Model file for the job. Use its own axes, mm. A direction names the side the tool comes from. Give positions to 0.01 mm unless a question says otherwise; leave off trailing zeros. Write each loop counter-clockwise with the first axis right and the second up, starting at its lowest first coordinate (ties: lowest second). Pieces come first, ordered by that corner, then holes. Notation, with made-up numbers: (73, 44) - (95, 44) arc R19 ccw to (95, 70) - close; hole circle Ø7 at (5, 52.5). An arc over 180 degrees is marked (long way). Use a Markdown table: item, result. Add a question column.
```python
from build123d import *

# Parameters (mm, degrees)
F1_DEPTH = 9
F2_R     = 5.5
F3_DEPTH = 51
F4_R     = 2.1
F5_DEPTH = 25
F6_R     = 5
F7_DEPTH = 25
F8_W     = 95
F8_H     = 11
F9_DEPTH = 25
F10_SIZE = 5
F11_SIZE = 2.1
F12_SIZE = 0.5


with BuildPart() as f1:
    # F0 (on Front) → F1 (new body, symmetric)
    with BuildSketch(Plane.XZ):
        Polygon((-245, 13.5), (-245, -37.5), (245, -37.5), (245, 13.5), (150, 13.5), (150, 37.5), (-150, 37.5), (-150, 13.5), align=None)
    extrude(amount=F1_DEPTH, both=True)

    # F2 (on face) → F3 (cut, through all)
    with BuildSketch(Plane(origin=(0, 0, -37.5), x_dir=(1, 0, 0), z_dir=(0, 0, -1))):
        with Locations((235, 0)):
            Circle(F2_R)
        with Locations((165, 0)):
            Circle(F2_R)
        with Locations((-165, 0)):
            Circle(F2_R)
        with Locations((-235, 0)):
            Circle(F2_R)
    extrude(amount=-F3_DEPTH, mode=Mode.SUBTRACT)

    # F4 (on face) → F5 (cut)
    with BuildSketch(Plane.XY.offset(37.5)):
        with Locations((-115, 0)):
            Circle(F4_R)
        with Locations((-55, 0)):
            Circle(F4_R)
        with Locations((5, 0)):
            Circle(F4_R)
        with Locations((65, 0)):
            Circle(F4_R)
        with Locations((125, 0)):
            Circle(F4_R)
    extrude(amount=-F5_DEPTH, mode=Mode.SUBTRACT)

    # F6 (on face) → F7 (cut)
    with BuildSketch(Plane.XY.offset(13.5)):
        with Locations((-200, 0)):
            Circle(F6_R)
        with Locations((200, 0)):
            Circle(F6_R)
    extrude(amount=-F7_DEPTH, mode=Mode.SUBTRACT)

    # F8 (on face) → F9 (cut)
    with BuildSketch(Plane.XZ.offset(9)):
        with Locations((-197.5, -32)):
            Rectangle(F8_W, F8_H)
        with Locations((197.5, -32)):
            Rectangle(F8_W, F8_H)
    extrude(amount=-F9_DEPTH, mode=Mode.SUBTRACT)

    # F10
    f10_edges = [f1.edges().sort_by_distance(p)[0] for p in [
        (-205, 0, -11.5),
        (195, 0, -11.5),
    ]]
    chamfer(f10_edges, length=F10_SIZE)

    # F11
    f11_edges = [f1.edges().sort_by_distance(p)[0] for p in [
        (122.9, 0, 12.5),
        (62.9, 0, 12.5),
        (2.9, 0, 12.5),
        (-57.1, 0, 12.5),
        (-117.1, 0, 12.5),
    ]]
    chamfer(f11_edges, length=F11_SIZE)

    # F12
    f12_edges = [f1.edges().sort_by_distance(p)[0] for p in [
        (-170.5, 0, -26.5),
        (-159.5, 0, -6.5),
        (-170.5, 0, 13.5),
        (-240.5, 0, -26.5),
        (-229.5, 0, -6.5),
        (-240.5, 0, 13.5),
        (-205, 0, 13.5),
        (-117.1, 0, 37.5),
        (-57.1, 0, 37.5),
        (2.9, 0, 37.5),
        (62.9, 0, 37.5),
        (122.9, 0, 37.5),
        (159.5, 0, -26.5),
        (170.5, 0, -6.5),
        (159.5, 0, 13.5),
        (229.5, 0, -26.5),
        (240.5, 0, -6.5),
        (229.5, 0, 13.5),
        (195, 0, 13.5),
    ]]
    chamfer(f12_edges, length=F12_SIZE)


solid = f1.part
```
(1) Band-saw the part on A-A (x = -165). Write the cut outline in (y, z), then the cut area to 4 significant figures.
(2) Which spindle directions (+Z, -Z, +X, -X, +Y, -Y) get a long thin tool onto all of the face, cutting with end or side? Do faces 1 (the cylindrical face through (204.77, 1.5, 3.39)), 2 (the flat face through (198, 6, 13.5)), 3 (the flat face through (-150, 0, -32)). Say none if no direction does.
(3) Flat gauge pins, fed straight in: pin 1 (9 mm diameter, centred on y = 4, z = 27.5, fed in from +X); pin 2 (6 mm diameter, centred on x = -164, y = 3.5, fed in from +Z); pin 3 (9 mm diameter, centred on y = -4.5, z = 26.5, fed in from -X). Where does each tip first touch, or does it go through?
(4) Probe probe 1 along X at (y, z) = (0, -18); probe 2 along Y at (x, z) = (-235, 2); probe 3 along Y at (x, z) = (65, 31.75). List the from-to ranges inside material, lowest first. Write a range as [from, to].
(5) Band-saw the part on B-B (z = 28.5). Write the cut outline in (x, y).
(6) Band-saw the part on C-C (z = -31.5). Write the cut outline in (x, y), then the cut area to 3 significant figures.
(7) Two-plate mould, pull along X, no slides. Class faces 4 (the cylindrical face through (159.505, -0.242, -6.773)), 5 (the flat face through (-3, -9, 1)), 6 (the flat face through (-150, 0, 26)): +X half, -X half, draft (parallel to the pull), parting line (faces both ways), or undercut.
Model answer:
| question | item | result |
|---|---|---|
| 1 | outline | (-9, -26.5) - (-6, -26.5) - (-5.5, -26) - (-5.5, 13) - (-6, 13.5) - (-9, 13.5) - close; (5.5, -26) - (6, -26.5) - (9, -26.5) - (9, 13.5) - (6, 13.5) - (5.5, 13) - close |
| 1 | area | 279.5 mm^2 |
| 2 | face 1 | +Z |
| 2 | face 2 | +Z, +X, +Y, -Y |
| 2 | face 3 | -Z, -X, +Y, -Y |
| 3 | pin 1 | stops at x = 150 |
| 3 | pin 2 | stops at z = 13.5 |
| 3 | pin 3 | stops at x = -150 |
| 4 | probe 1 | x = [-245, -240.5], [-229.5, -170.5], [-159.5, 159.5], [170.5, 229.5], [240.5, 245] |
| 4 | probe 2 | y = [-9, -5.5], [5.5, 9] |
| 4 | probe 3 | y = [-9, -2.1], [2.1, 9] |
| 5 | outline | (-150, -9) - (150, -9) - (150, 9) - (-150, 9) - close; hole circle Ø4.2 at (-115, 0); hole circle Ø4.2 at (-55, 0); hole circle Ø4.2 at (5, 0); hole circle Ø4.2 at (65, 0); hole circle Ø4.2 at (125, 0) |
| 6 | outline | (-150, -9) - (150, -9) - (150, 9) - (-150, 9) - close |
| 6 | area | 5,400 mm^2 |
| 7 | face 4 | undercut |
| 7 | face 5 | draft |
| 7 | face 6 | -X half |
